CAD build for the part. Positions are in the model's coordinates, mm. A direction names the side the tool comes from. Give positions to 0.01 mm unless a question says otherwise; leave off trailing zeros. Loops run counter-clockwise (first coordinate to the right, second up) from the corner with the lowest first, then second, coordinate; pieces in that order, holes last. Notation, with made-up numbers: M 49,-12 L 65,-12 A30 cw 65,20 Z; hole C 2,83 d11. An arc over 180 degrees is marked long. Answer as CSV lines item,"result".
Autodesk Fusion 360 part; units mm, degrees
sketch "Roller_End_Cap_Outter" plane through (0, 0, 0) normal (0, 0, 1) x (1, 0, 0)
  circle A0 centre (0, 0) radius 38.1
  dimension "d2" = 76.2
extrude "Extrude1" add sketch "Roller_End_Cap_Outter" along normal blind 6.35
sketch "Roller_End_Cap_Inner" plane through (0, 0, 6.35) normal (0, 0, 1) x (-1, 0, 0)
  circle A0 centre (0, 0) radius 38.1
  circle A1 centre (0, 0) radius 34.925
  dimension "d7" = 69.85
extrude "Extrude3" add sketch "Roller_End_Cap_Inner" along normal blind 10 contours A1
sketch "Shaft Hole" plane through (0, 0, 16.35) normal (0, 0, 1) x (-1, 0, 0)
  circle A0 centre (0, 0) radius 34.925
  circle A1 centre (0, 0) radius 6.45
  dimension "d10" = 12.9
extrude "Extrude4" cut sketch "Shaft Hole" against normal through all contours A1
extrude "Extrude5" add 1 faces at (-25.3033, 1.7351, 16.35) along direction (0, 0, 1) blind 3.65
chamfer "Chamfer1" distance 2 angle 45 1 edges at (6.0135, -2.3324, 20)
chamfer "Chamfer2" distance 2 angle 45 1 edges at (32.5615, 12.6294, 20)
Q1. Pin check, flat tips, straight feed: P1, Ø6, axis at x = 11.5, z = 12.5, coming from the -Y side; P2, Ø1, axis at y = -14, z = 15, coming from the +X side; P3, Ø12, axis at x = -19.5, z = 14, coming from the -Y side. Stop position of each tip, or through.
Solution:
P1,"stops at y = -33.87"
P2,"stops at x = 32.21"
P3,"stops at y = -32.21"
Q2. Cut at A-A (y = 0). Write the cut outline in (x, z) (3 decimals), and give its area (3 significant figures).
Solution:
outline,"M -38.1,0 L -6.45,0 L -6.45,18 L -8.45,20 L -32.925,20 L -34.925,18 L -34.925,6.35 L -38.1,6.35 Z; M 6.45,0 L 38.1,0 L 38.1,6.35 L 34.925,6.35 L 34.925,18 L 32.925,20 L 8.45,20 L 6.45,18 Z"
area,"1,170 mm²"
Q3. Which spindle directions (+Z, -Z, +X, -X, +Y, -Y) get a long thin tool onto all of the face, cutting with end or side? Do faces 1 (the cylindrical face through (27.715, -21.251, 12.093)), 2 (the flat face through (8, 1, 0)). Say none if no direction does.
Solution:
face 1,"+Z"
face 2,"-Z, +X, -X, +Y, -Y"
Q4. Mould opens along Y. For faces 3 (the conical face through (-15.251, -29.321, 19.875)), 4 (the flat face through (-7, 7, 20)), 5 (the cylindrical face through (1.398, -6.297, 8.874)) say: released by +Y, released by -Y, zero draft, split by the parting line, or undercut.
Solution:
face 3,"split by the parting line"
face 4,"zero draft"
face 5,"undercut"
Q5. Wall check: line 1 (Y direction, x = 0, z = 9) (3 decimals); line 2 (Y direction, x = -5, z = 18.25). Give the ranges that are in metal, low to high. Write a range as [from, to].
Solution:
line 1,"y = [-34.925, -6.45], [6.45, 34.925]"
line 2,"y = [-34.31, -4.46], [4.46, 34.31]"
Q6. Cut at C-C (z = 10.5). Write the cut outline in (x, y) (3 decimals), and give its area (3 significant figures).
Solution:
outline,"C 0,0 d69.85; hole C 0,0 d12.9"
area,"3,700 mm²"
